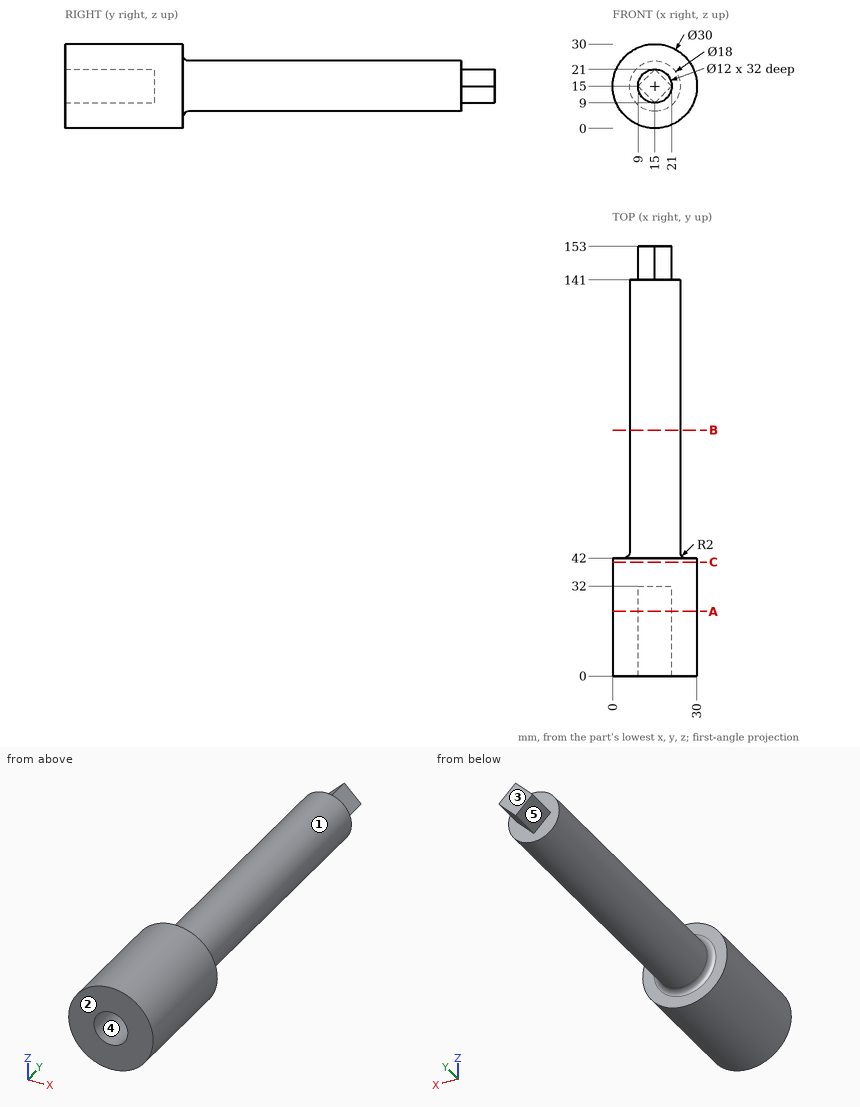
For this review, use the dimensioned drawing (mm, ordinates from the lowest corner) and the shaded views. A direction names the side the tool comes from. Give positions to 0.01 mm unless a question says otherwise; leave off trailing zeros. Order: outer loops, then holes, each group sorted by start corner. A loop starts at its lowest first (then second) coordinate and runs counter-clockwise, first axis right, second up. Notation, with made-up numbers: (5, 71.25) - (19, 71.25) arc R20 ccw to (19, 75.25) - close; hole circle Ø4 at (40.25, 24). An arc over 180 degrees is marked (long way). Write item = value, one per line. Start each with the question number.
Q1. Mouldability with a two-part tool opening along Z and no side actions: class the marked faces 3, 4 and 5 as released by +Z, released by -Z, zero draft, split by the parting line, or undercut.
Q2. We need section C-C on y = 40.5. State the section outline as (x, z) points, plus the area to 3 significant figures.
Q3. We need section A-A on y = 23. State the section outline as (x, z) points, plus the area to 3 significant figures.
Q4. Tool access review of the marked faces 1 and 2: name each direction out of +Z, -Z, +X, -X, +Y, -Y from which nothing blocks a thin tool from reaching the whole face with its end or side.
Q5. Clearance check with flat-ended pins moving along their axes: pin 1 Ø12 at (y, z) = (22.5, 16) entering from +X; pin 2 Ø10 at (x, y) = (23, 137) entering from -Z; pin 3 Ø11 at (x, z) = (15, 15) entering from -Y; pin 4 Ø4 at (x, y) = (12, 101) entering from -Z. State where each tip first meets the part, or that it passes through.
Q6. We need section B-B on y = 87.5. State the section outline as (x, z) points.
Q7. To check wall thickness, follow L1, parallel to X at y = 21, z = 15; L2, parallel to Y at x = 19.75, z = 27; L3, parallel to Y at x = 22.25, z = 14.25. State the ranges of each line that lie inside material, in increasing order. Write a range as from..to.
Working result:
q1.face_3 = zero draft
q1.face_4 = undercut
q1.face_5 = released by -Z
q2.outline = circle Ø30 at (15, 15)
q2.area = 707 mm²
q3.outline = circle Ø30 at (15, 15); hole circle Ø12 at (15, 15)
q3.area = 594 mm²
q4.face_1 = +Y
q4.face_2 = +Z, -Z, +X, -X, -Y
q5.pin_1 = 30
q5.pin_2 = 6.51
q5.pin_3 = 32
q5.pin_4 = 6.06
q6.outline = circle Ø18 at (15, 15)
q7.L1 = 0..9, 21..30
q7.L2 = 0..42
q7.L3 = 0..141
